```python
from build123d import *

# Parameters (mm, degrees)
SKETCH1_W                       = 11
SKETCH1_H                       = 11
BOSS_EXTRUDE1_DEPTH             = 8
BOSS_EXTRUDE2_REACH             = 16
SKETCH2_W                       = 3
SKETCH2_H                       = 5
FILLET1_R                       = 3
M5_TAPPED_HOLE1_D               = 4.2
M5_TAPPED_HOLE1_DEPTH           = 4
M5_TAPPED_HOLE1_ON_FACE_2_D     = 4.2
M5_TAPPED_HOLE1_ON_FACE_2_DEPTH = 4


with BuildPart() as part:
    # Sketch1 → Boss-Extrude1 (new body)
    with BuildSketch(Plane.XY):
        with BuildLine():
            Line((50, -5.203998401), (50, -14))
            ThreePointArc((50, -14), (48.535533906, -17.535533906), (45, -19))
            Line((45, -19), (-45, -19))
            ThreePointArc((-45, -19), (-48.535533906, -17.535533906), (-50, -14))
            Line((-50, -14), (-50, -5.203998401))
            ThreePointArc((-50, -5.203998401), (-48.46415928, -1.59850253), (-44.800159808, -0.207993608))
            Line((-44.800159808, -0.207993608), (0, -2))
            Line((0, -2), (44.800159808, -0.207993608))
            ThreePointArc((44.800159808, -0.207993608), (48.46415928, -1.59850253), (50, -5.203998401))
        make_face()
        with Locations((-40.5, -9.5)):
            Rectangle(SKETCH1_W, SKETCH1_H, mode=Mode.SUBTRACT)
        with Locations((40.5, -9.5)):
            Rectangle(SKETCH1_W, SKETCH1_H, mode=Mode.SUBTRACT)
        with BuildLine():
            Line((-25, -5), (25, -5))
            ThreePointArc((25, -5), (30, -10), (25, -15))
            Line((25, -15), (-25, -15))
            ThreePointArc((-25, -15), (-30, -10), (-25, -5))
        make_face(mode=Mode.SUBTRACT)
    extrude(amount=BOSS_EXTRUDE1_DEPTH)

    # Sketch2 → Boss-Extrude2 (add, up to next)
    with BuildSketch(Plane.XZ.offset(5), mode=Mode.PRIVATE) as boss_extrude2_sk1:
        with Locations((-9.5, 2.5)):
            Rectangle(SKETCH2_W, SKETCH2_H)
    boss_extrude2_tool1 = extrude(boss_extrude2_sk1.sketch, amount=BOSS_EXTRUDE2_REACH, mode=Mode.PRIVATE) - part.part
    add(boss_extrude2_tool1.solids().sort_by_distance((-9.5, -5, 2.5))[0])
    # Sketch2 → Boss-Extrude2 (add, up to next)
    with BuildSketch(Plane.XZ.offset(5), mode=Mode.PRIVATE) as boss_extrude2_sk2:
        with Locations((9.5, 2.5)):
            Rectangle(SKETCH2_W, SKETCH2_H)
    boss_extrude2_tool2 = extrude(boss_extrude2_sk2.sketch, amount=BOSS_EXTRUDE2_REACH, mode=Mode.PRIVATE) - part.part
    add(boss_extrude2_tool2.solids().sort_by_distance((9.5, -5, 2.5))[0])

    # Fillet1
    fillet1_edges = [part.edges().sort_by_distance(p)[0] for p in [
        (-8, -15, 2.5),
        (-8, -5, 2.5),
        (-11, -15, 2.5),
        (-11, -5, 2.5),
        (11, -15, 2.5),
        (11, -5, 2.5),
        (8, -15, 2.5),
        (8, -5, 2.5),
    ]]
    fillet(fillet1_edges, radius=FILLET1_R)

    # M5 Tapped Hole1
    with Locations(Plane(origin=(-50, -9.703998401, 4), x_dir=(0, 0, -1), z_dir=(-1, 0, 0))):
        with Locations((0, 0)):
            Hole(M5_TAPPED_HOLE1_D / 2, depth=M5_TAPPED_HOLE1_DEPTH)

    # M5 Tapped Hole1 on face 2
    with Locations(Plane(origin=(50, -9.703998401, 4), x_dir=(0, 0, 1), z_dir=(1, 0, 0))):
        with Locations((0, 0)):
            Hole(M5_TAPPED_HOLE1_ON_FACE_2_D / 2, depth=M5_TAPPED_HOLE1_ON_FACE_2_DEPTH)


solid = part.part
```
Geometry: final body of the model. Coordinates: model frame, mm. A direction names the side the tool comes from. Round coordinates to 2 decimals unless told otherwise and drop trailing zeros. Order: outer loops, then holes, each group sorted by start corner. A loop starts at its lowest first (then second) coordinate and runs counter-clockwise, first axis right, second up. Notation, with made-up numbers: (31.25, 16.25) -> (68.25, 16.25) arc R28 cw to (68.25, 42.25) -> close; hole circle Ø11 at (-8.75, 22.5). An arc over 180 degrees is marked (long way). Write each question's results on one line, items separated by ' | '.
Q1. Section query D-D (z = 4). Count the separate pieces of the cut face and the enclosed holes in it, and give its area (3 significant figures).
Response values:
separate pieces: 1 | enclosed holes: 3 | area: 999 mm²
Q2. Ray query, line 1 along X through (y, z) = (-8.25, 1.75); line 2 along Y through (x, z) = (45, 4.5); line 3 along X through (y, z) = (-13, 1.75). Return the intervals inside material, ascending.
Response values:
line 1: -50 to -46, -35 to -29.68, -11 to -8, 8 to 11, 29.68 to 35, 46 to 50 | line 2: -19 to -15, -4 to -0.2 | line 3: -50 to -46, -35 to -29, -11.17 to -7.83, 7.83 to 11.17, 29 to 35, 46 to 50
Q3. Section query A-A (x = -18). Output: boundary loops of the cut face in (y, z).
Response values:
outline: (-19, 0) -> (-15, 0) -> (-15, 8) -> (-19, 8) -> close; (-5, 0) -> (-1.28, 0) -> (-1.28, 8) -> (-5, 8) -> close
Q4. Access query for faces 4 (the face through (49, -17, 4)), 5 (the face through (0, -15, 5)), 6 (the face through (46, -8, 2)). Directions: +Z, -Z, +X, -X, +Y, -Y. A direction counts if a zero-diameter tool reaches every point of the face in a straight line with its end or side. Return the directions, or none.
Response values:
face 4: +Z, -Z, +X, -Y | face 5: +Z | face 6: +Z, -Z
Q5. Pull-direction query (Y, two-part tool) for faces 1 (the face through (-22.71, -1.09, 3.94)), 2 (the face through (-11.9, -14.14, 2.54)), 3 (the face through (-50, -12, 3)); classes: released by +Y, released by -Y, zero draft, split by the parting line, or undercut.
Response values:
face 1: released by +Y | face 2: undercut | face 3: zero draft
Q6. Section query C-C (y = -13). Output: boundary loops of the cut face in (x, z).
Response values:
outline: (-50, 0) -> (-46, 0) -> (-46, 8) -> (-50, 8) -> close; (-35, 0) -> (-29, 0) -> (-29, 8) -> (-35, 8) -> close; (-11.17, 0) -> (-7.83, 0) -> (-7.83, 5) -> (-11.17, 5) -> close; (7.83, 0) -> (11.17, 0) -> (11.17, 5) -> (7.83, 5) -> close; (29, 0) -> (35, 0) -> (35, 8) -> (29, 8) -> close; (46, 0) -> (50, 0) -> (50, 8) -> (46, 8) -> close
Q7. Pin query (flat end, axial travel): pin 1 Ø4 at (x, z) = (42.5, 3) entering from +Y; pin 2 Ø4 at (x, z) = (-39, 3.5) entering from +Y. Return the tip coordinate at first contact, or that it passes through.
Response values:
pin 1: y = -0.22 | pin 2: y = -0.36
Q8. Section query B-B (x = -3.5). Output: boundary loops of the cut face in (y, z), and give its area (3 significant figures).
Response values:
outline: (-19, 0) -> (-15, 0) -> (-15, 8) -> (-19, 8) -> close; (-5, 0) -> (-1.86, 0) -> (-1.86, 8) -> (-5, 8) -> close | area: 57.1 mm²
